For this review, take the finished solid that the model builds, in its own axes (mm). A direction names the side the tool comes from. Give positions to 0.01 mm unless a question says otherwise; leave off trailing zeros. Loops run counter-clockwise (first coordinate to the right, second up) from the corner with the lowest first, then second, coordinate; pieces in that order, holes last. Notation, with made-up numbers: (-36, -6) - (-17, -6) arc R19 cw to (-17, 1) - close; hole circle Ø4 at (-38, -29). An arc over 180 degrees is marked (long way). Answer as CSV lines item,"result".
from build123d import *

# Parameters (mm, degrees)
F0_W     = 30
F0_H     = 15
F0_R     = 1.5
F1_DEPTH = 2
F2_W     = 30
F2_H     = 3
F3_DEPTH = 35
F4_SIZE  = 25
F6_D     = 2.5


with BuildPart() as f1:
    # F0 (on Top) → F1 (new body)
    with BuildSketch(Plane.XY):
        Rectangle(F0_W, F0_H)
        with Locations((-7.5, -4.5)):
            Circle(F0_R, mode=Mode.SUBTRACT)
        with Locations((0, -4.5)):
            Circle(F0_R, mode=Mode.SUBTRACT)
        with Locations((7.5, -4.5)):
            Circle(F0_R, mode=Mode.SUBTRACT)
        with Locations((-7.5, 4.5)):
            Circle(F0_R, mode=Mode.SUBTRACT)
        with Locations((0, 4.5)):
            Circle(F0_R, mode=Mode.SUBTRACT)
        with Locations((7.5, 4.5)):
            Circle(F0_R, mode=Mode.SUBTRACT)
    extrude(amount=F1_DEPTH)

    # F2 (on face) → F3 (join)
    with BuildSketch(Plane.XY.offset(2)):
        Rectangle(F2_W, F2_H)
    extrude(amount=F3_DEPTH)

    # F4
    f4_edges = [f1.edges().sort_by_distance(p)[0] for p in [
        (-15, 0, 37),
    ]]
    chamfer(f4_edges, length=F4_SIZE)

    # F6 (through all)
    with Locations(Plane.XZ.offset(1.5)):
        with Locations((12.5, 32), (12.5, 27), (12.5, 22), (12.5, 17), (12.5, 12)):
            Hole(F6_D / 2)


solid = f1.part
1) Machinability: for faces 5 (the cylindrical face through (13.421, 0.021, 27.845)), 6 (the flat face through (0, -2, 2)), 7 (the flat face through (3, 1.5, 15)), which of the approach directions +Z, -Z, +X, -X, +Y, -Y give a long, thin tool a straight path to every point of the face, cutting with its end or side? Answer none if there is none.
From the geometry:
face 5,"+Y, -Y"
face 6,"+Z, +X, -X, -Y"
face 7,"+Z, +X, -X, +Y"
2) Wall thickness on line 1 (Y direction, x = 0, z = 0.9); line 2 (Y direction, x = 3.5, z = 18.5); line 3 (X direction, y = 0.5, z = 30): over which ranges is each line inside the solid? List them lowest first. Write a range as from..to.
From the geometry:
line 1,"y = -7.5..-6, -3..3, 6..7.5"
line 2,"y = -1.5..1.5"
line 3,"x = 3..15"
3) Consider section D-D on x = -3.25. Write out the cut boundary in (y, z), and give its area (4 significant figures).
From the geometry:
outline,"(-7.5, 0) - (7.5, 0) - (7.5, 2) - (1.5, 2) - (1.5, 23.75) - (-1.5, 23.75) - (-1.5, 2) - (-7.5, 2) - close"
area,"95.25 mm^2"
4) Draft analysis for pull direction X (two halves, no side actions). For faces 1 (the flat face through (3, -1.5, 15)), 2 (the flat face through (-15, 0, 4)), 3 (the cylindrical face through (6, 4.57, 0.99)), 4 (the cylindrical face through (-9, -4.43, 0.99)), state which applies: pulls with the +X half, pulls with the -X half, needs draft (parallel to the pull), parting line crosses it, or undercut.
From the geometry:
face 1,"needs draft"
face 2,"pulls with the -X half"
face 3,"undercut"
face 4,"undercut"
5) Consider section C-C on y = 0. Write out the cut boundary in (x, z), and give its area (3 significant figures).
From the geometry:
outline,"(-15, 0) - (15, 0) - (15, 37) - (10, 37) - (-15, 12) - close; hole circle Ø2.5 at (12.5, 12); hole circle Ø2.5 at (12.5, 17); hole circle Ø2.5 at (12.5, 22); hole circle Ø2.5 at (12.5, 27); hole circle Ø2.5 at (12.5, 32)"
area,"773 mm^2"
6) Consider section A-A on z = 27. Write out the cut boundary in (x, y).
From the geometry:
outline,"(0, -1.5) - (11.25, -1.5) - (11.25, 1.5) - (0, 1.5) - close; (13.75, -1.5) - (15, -1.5) - (15, 1.5) - (13.75, 1.5) - close"
7) Insertion check: P1, Ø4, axis at x = 12.5, z = 17, coming from the -Y side; P2, Ø6.5, axis at x = 6.5, y = -5, coming from the +Z side; P3, Ø5, axis at x = 6.5, y = -4, coming from the -Z side; P4, Ø1, axis at x = -4, z = 21.5, coming from the +Y side. Each pin has a flat end and moves straight along its axis. Give the tip position at first contact, or say it passes through.
From the geometry:
P1,"stops at y = -1.5"
P2,"stops at z = 2"
P3,"stops at z = 0"
P4,"stops at y = 1.5"
8) Consider section B-B on x = 12.5. Write out the cut boundary in (y, z), and give its area (3 significant figures).
From the geometry:
outline,"(-7.5, 0) - (7.5, 0) - (7.5, 2) - (1.5, 2) - (1.5, 10.75) - (-1.5, 10.75) - (-1.5, 2) - (-7.5, 2) - close; (-1.5, 13.25) - (1.5, 13.25) - (1.5, 15.75) - (-1.5, 15.75) - close; (-1.5, 18.25) - (1.5, 18.25) - (1.5, 20.75) - (-1.5, 20.75) - close; (-1.5, 23.25) - (1.5, 23.25) - (1.5, 25.75) - (-1.5, 25.75) - close; (-1.5, 28.25) - (1.5, 28.25) - (1.5, 30.75) - (-1.5, 30.75) - close; (-1.5, 33.25) - (1.5, 33.25) - (1.5, 37) - (-1.5, 37) - close"
area,"97.5 mm^2"
